```python
from build123d import *

# Parameters (mm, degrees)
F1_DEPTH = 12.7
F2_W     = 43.1732637808
F2_H     = 15.9647427499
F3_DEPTH = 12.7
F4_W     = 61.8251115084
F4_H     = 15.9647427499
F5_DEPTH = 76.2
F7_DEPTH = 25.4


with BuildPart() as f1:
    # F0 (on Top) → F1 (new body)
    with BuildSketch(Plane.XY):
        with BuildLine():
            Line((13.5834803805, 41.8586246669), (-29.5897834003, 41.8586246669))
            Line((-29.5897834003, 41.8586246669), (-29.5897834003, -19.0352704376))
            Line((-29.5897834003, -19.0352704376), (-29.5897834003, -39.5325236022))
            ThreePointArc((-29.5897834003, -39.5325236022), (-0.4357211292, -54.9443437525), (28.7183411419, -39.5325236022))
            Line((28.7183411419, -39.5325236022), (28.7183411419, -19.0352704376))
            Line((28.7183411419, -19.0352704376), (13.5834803805, -19.0352704376))
            Line((13.5834803805, -19.0352704376), (13.5834803805, 41.8586246669))
        make_face()
    extrude(amount=F1_DEPTH)

    # F2 (on face) → F3 (join)
    with BuildSketch(Plane.XY.offset(12.7)):
        with Locations((-8.0031515099, 33.876253292)):
            Rectangle(F2_W, F2_H)
    extrude(amount=F3_DEPTH)

    # F4 (on face) → F5 (join)
    with BuildSketch(Plane.XY.offset(25.4)):
        with Locations((1.3227723539, 33.876253292)):
            Rectangle(F4_W, F4_H)
    extrude(amount=F5_DEPTH)

    # F6 (on face) → F7 (cut)
    with BuildSketch(Plane.XZ.offset(-25.893881917)):
        with BuildLine():
            Line((11.6920806468, 101.6), (-8.112533018, 101.6))
            Line((-8.112533018, 101.6), (-8.112533018, 51.0209538043))
            ThreePointArc((-8.112533018, 51.0209538043), (1.7897738144, 41.1186469719), (11.6920806468, 51.0209538043))
            Line((11.6920806468, 51.0209538043), (11.6920806468, 101.6))
        make_face()
    extrude(amount=-F7_DEPTH, mode=Mode.SUBTRACT)


solid = f1.part
```
Check sheet for the modelled part. Datum: model origin and axes. Units: mm. A direction names the side the tool comes from. Coordinates: 2 decimals unless noted, no trailing zeros. Order: outer loops, then holes, each group sorted by start corner. A loop starts at its lowest first (then second) coordinate and runs counter-clockwise, first axis right, second up. Notation, with made-up numbers: (-10, 33.25) -> (24, 33.25) arc R7 cw to (24, 39.25) -> close; hole circle Ø10 at (-38, -13.5). An arc over 180 degrees is marked (long way). Write item = value, one per line. Start each with the question number.
1) Cross-section at B-B (y = 35.5). Enter the section's corners in (x, z), then the cut area to 3 significant figures.
2) Cross-section at D-D (x = -3). Enter the section's corners in (y, z).
3) Material ranges on L1, parallel to X at y = 27.5, z = 81; L2, parallel to X at y = 17.5, z = 5; L3, parallel to Z at x = 18.5, y = -26.5, recorded low to high.
4) Cross-section at C-C (x = 15). Enter the section's corners in (y, z), then the cut area to 3 significant figures.
5) Cross-section at A-A (z = 78.5). Enter the section's corners in (x, y).
6) Access from +Z, -Z, +X, -X, +Y, -Y to the whole of each face (thin tool, end or side, straight path). Record for faces 1 (the flat face through (23, 34, 25.4)), 2 (the flat face through (-7, -14, 12.7)), 3 (the flat face through (-8.113, 34, 77)), 4 (the flat face through (13.583, 18, 10)).
7) Mould release check, pull along X, two halves, no side actions. Record for faces 5 (the cylindrical face through (1.57, 33.76, 41.12)), 6 (the flat face through (11.692, 34, 76)), 7 (the flat face through (21, -19.035, 6)), 8 (the flat face through (-29.59, 28, 36)): +X half, -X half, draft (parallel to the pull), parting line (faces both ways), or undercut.
8) Go/stop test with flat-tipped pins: P1, Ø10, axis at x = -2, z = 14.5, coming from the -Y side; P2, Ø10, axis at x = 23.5, z = 6, coming from the +Y side; P3, Ø3, axis at x = -22.5, y = 7, coming from the +Z side. Record where each tip stops, or that it passes through.
Ans:
q1.outline = (-29.59, 0) -> (13.58, 0) -> (13.58, 25.4) -> (32.24, 25.4) -> (32.24, 101.6) -> (11.69, 101.6) -> (11.69, 51.02) arc R9.9 cw to (-8.11, 51.02) -> (-8.11, 101.6) -> (-29.59, 101.6) -> close
q1.area = 4,650 mm²
q2.outline = (-54.85, 0) -> (41.86, 0) -> (41.86, 42.35) -> (25.89, 42.35) -> (25.89, 12.7) -> (-54.85, 12.7) -> close
q3.L1 = -29.59 to -8.11, 11.69 to 32.24
q3.L2 = -29.59 to 13.58
q3.L3 = 0 to 12.7
q4.outline = (-51.39, 0) -> (-19.04, 0) -> (-19.04, 12.7) -> (-51.39, 12.7) -> close; (25.89, 25.4) -> (41.86, 25.4) -> (41.86, 101.6) -> (25.89, 101.6) -> close
q4.area = 1,630 mm²
q5.outline = (-29.59, 25.89) -> (-8.11, 25.89) -> (-8.11, 41.86) -> (-29.59, 41.86) -> close; (11.69, 25.89) -> (32.24, 25.89) -> (32.24, 41.86) -> (11.69, 41.86) -> close
q6.face_1 = -Z, +X, +Y, -Y
q6.face_2 = +Z, +X, -X, -Y
q6.face_3 = +Z, +Y, -Y
q6.face_4 = -Z, +X, +Y
q7.face_5 = undercut
q7.face_6 = undercut
q7.face_7 = draft
q7.face_8 = -X half
q8.P1 = -54.94
q8.P2 = -19.04
q8.P3 = 12.7
